Geometry check sheet. Reference: the model listing, model coordinates, mm. Round coordinates to 2 decimals unless told otherwise and drop trailing zeros. Write each loop counter-clockwise with the first axis right and the second up, starting at its lowest first coordinate (ties: lowest second). Pieces come first, ordered by that corner, then holes. Notation, with made-up numbers: M 2,67 L 16,67 A13 cw 16,76 Z; hole C -26.75,-9 d2. An arc over 180 degrees is marked long. One line per item, written item: value. Start each with the question number.
1. Scan lines: probe 1 along X at (y, z) = (1.35, -32.5); probe 2 along Z at (x, y) = (-15, 2.1); probe 3 along X at (y, z) = (4.45, -32.5). Record each from-to range of solid material in increasing order. Write a range as [from, to].
2. Section check D-D (x = 14.5). Record the boundary of the cut face in (y, z), and give its area (3 significant figures).
3. Section check C-C (y = 1.5). Record the boundary of the cut face in (x, z), and give its area (3 significant figures).
4. Section check B-B (x = -15). Record the boundary of the cut face in (y, z).
5. Section check A-A (z = 0). Record the boundary of the cut face in (x, y).
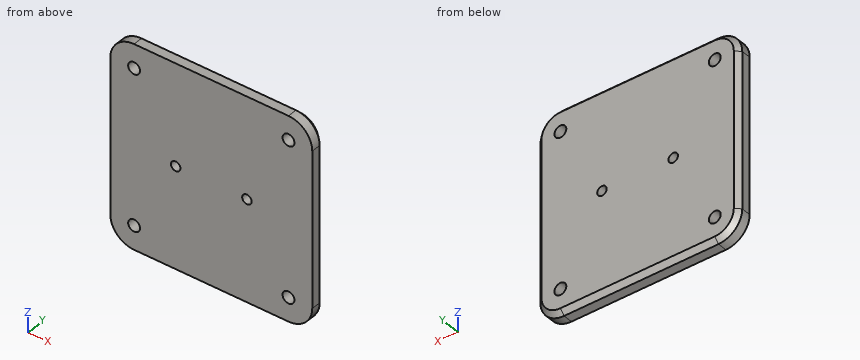
from build123d import *

# Parameters (mm, degrees)
SKETCH1_R                 = 2.5
BOSS_EXTRUDE1_DEPTH       = 6
CHAMFER1_SIZE             = 2
M4X0_7_TAPPED_HOLE2_D     = 4
M4X0_7_TAPPED_HOLE2_DEPTH = 8.898278762
M4X0_7_TAPPED_HOLE2_TIP   = 1.201721238


with BuildPart() as part:
    # Sketch1 → Boss-Extrude1 (new body)
    with BuildSketch(Plane(origin=(0, 0, 0), x_dir=(1, 0, 0), z_dir=(0, 1, 0))):
        with BuildLine():
            Line((-32.5, -42.5), (32.5, -42.5))
            ThreePointArc((32.5, -42.5), (39.571067812, -39.571067812), (42.5, -32.5))
            Line((42.5, -32.5), (42.5, 32.5))
            ThreePointArc((42.5, 32.5), (39.571067812, 39.571067812), (32.5, 42.5))
            Line((32.5, 42.5), (-32.5, 42.5))
            ThreePointArc((-32.5, 42.5), (-39.571067812, 39.571067812), (-42.5, 32.5))
            Line((-42.5, 32.5), (-42.5, -32.5))
            ThreePointArc((-42.5, -32.5), (-39.571067812, -39.571067812), (-32.5, -42.5))
        make_face()
        with Locations(Location((-32.5, 32.5, 0), (0, 0, 270))):
            Circle(SKETCH1_R, mode=Mode.SUBTRACT)
        with Locations(Location((32.5, 32.5, 0), (0, 0, 90))):
            Circle(SKETCH1_R, mode=Mode.SUBTRACT)
        with Locations(Location((32.5, -32.5, 0), (0, 0, 270))):
            Circle(SKETCH1_R, mode=Mode.SUBTRACT)
        with Locations(Location((-32.5, -32.5, 0), (0, 0, 90))):
            Circle(SKETCH1_R, mode=Mode.SUBTRACT)
    extrude(amount=BOSS_EXTRUDE1_DEPTH)

    # Chamfer1
    chamfer1_edges = [part.edges().sort_by_distance(p)[0] for p in [
        (39.571067812, 6, -39.571067812),
        (42.5, 6, 0),
        (39.571067812, 6, 39.571067812),
        (0, 6, 42.5),
        (-39.571067812, 6, 39.571067812),
    ]]
    chamfer(chamfer1_edges, length=CHAMFER1_SIZE)

    # M4x0.7 Tapped Hole2
    with Locations(Plane(origin=(0, 6, 0), x_dir=(1, 0, 0), z_dir=(0, 1, 0))):
        with Locations((-15, 0), (15, 0)):
            Hole(M4X0_7_TAPPED_HOLE2_D / 2, depth=M4X0_7_TAPPED_HOLE2_DEPTH)
            with Locations((0, 0, -(M4X0_7_TAPPED_HOLE2_DEPTH + M4X0_7_TAPPED_HOLE2_TIP / 2))):  # 118° drill point
                Cone(0, M4X0_7_TAPPED_HOLE2_D / 2, M4X0_7_TAPPED_HOLE2_TIP, mode=Mode.SUBTRACT)


solid = part.part
Result sheet:
1. probe 1: x = [-42.5, -35], [-30, 30], [35, 42.5]
1. probe 2: z = [-42.5, -2], [2, 42.5]
1. probe 3: x = [-42.05, -35], [-30, 30], [35, 42.05]
2. outline: M 0,-42.5 L 4,-42.5 L 6,-40.5 L 6,-1.94 L 0,-1.94 Z; M 0,1.94 L 6,1.94 L 6,40.5 L 4,42.5 L 0,42.5 Z
2. area: 483 mm2
3. outline: M -42.5,-32.5 A10 ccw -32.5,-42.5 L 32.5,-42.5 A10 ccw 42.5,-32.5 L 42.5,32.5 A10 ccw 32.5,42.5 L -32.5,42.5 A10 ccw -42.5,32.5 Z; hole C -32.5,-32.5 d5; hole C -32.5,32.5 d5; hole C -15,0 d4; hole C 15,0 d4; hole C 32.5,-32.5 d5; hole C 32.5,32.5 d5
3. area: 7,040 mm2
4. outline: M 0,-42.5 L 4,-42.5 L 6,-40.5 L 6,-2 L 0,-2 Z; M 0,2 L 6,2 L 6,40.5 L 4,42.5 L 0,42.5 Z
5. outline: M -42.5,0 L -17,0 L -17,6 L -40.5,6 L -42.5,4 Z; M -13,0 L 13,0 L 13,6 L -13,6 Z; M 17,0 L 42.5,0 L 42.5,4 L 40.5,6 L 17,6 Z
